from build123d import *

# Parameters (mm, degrees)
BOSS_EXTRUDE1_DEPTH      = 5
BOSS_EXTRUDE1_DEPTH_BACK = 10
SKETCH1_R                = 12.5


with BuildPart() as part:
    # Sketch1 → Boss-Extrude1 (new, two sides: drawn at the far end of the back side and taken through both)
    with BuildSketch(Plane.XY.offset(-BOSS_EXTRUDE1_DEPTH_BACK)):
        with BuildLine():
            Line((-44.88915592, -28.254421038), (-43.965658713, -46.45807859))
            ThreePointArc((-43.965658713, -46.45807859), (-28.965658713, -61.45807859), (-13.965658713, -46.45807859))
            Line((-13.965658713, -46.45807859), (-14.042670787, -44.940043234))
            Line((-14.042670787, -44.940043234), (-14.968304337, -26.694274815))
            ThreePointArc((-14.968304337, -26.694274815), (-29.72001982, -31.477043366), (-44.88915592, -28.254421038))
        make_face()
        with Locations((-28.965658713, -46.45807859)):
            Circle(SKETCH1_R, mode=Mode.SUBTRACT)
    extrude(amount=BOSS_EXTRUDE1_DEPTH + BOSS_EXTRUDE1_DEPTH_BACK)


solid = part.part
The listing builds one solid part. Answer for the finished solid, in the listing's coordinates (mm). Give positions to 0.01 mm unless a question says otherwise; leave off trailing zeros. Write each loop counter-clockwise with the first axis right and the second up, starting at its lowest first coordinate (ties: lowest second). Pieces come first, ordered by that corner, then holes. Notation, with made-up numbers: (16.5, -38) - (73.5, -38) arc R14 cw to (73.5, -27) - close; hole circle Ø11 at (32.25, 75.5). An arc over 180 degrees is marked (long way). Use a Markdown table: item, result.
1. Section C-C on y = -46 is taken. Write down the section's boundary in (x, z), plus the area to 3 significant figures.
Values follow:
| item | result |
|---|---|
| outline | (-43.99, -10) - (-41.46, -10) - (-41.46, 5) - (-43.99, 5) - close; (-16.47, -10) - (-13.99, -10) - (-13.99, 5) - (-16.47, 5) - close |
| area | 75.3 mm² |
2. For a pull along X with two mould halves and no side action, classify faces 1 (the cylindrical face through (-29.501, -31.465, -2.605)), 2 (the cylindrical face through (-22.246, -35.918, -2.605)), 3 (the flat face through (-37, -36, -10)), 4 (the cylindrical face through (-29.295, -61.454, -2.605)) as released by +X, released by -X, zero draft, split by the parting line, or undercut.
Values follow:
| item | result |
|---|---|
| face 1 | undercut |
| face 2 | undercut |
| face 3 | zero draft |
| face 4 | split by the parting line |
3. Section A-A on x = -37 is taken. Write down the section's boundary in (y, z), plus the area to 3 significant figures.
Values follow:
| item | result |
|---|---|
| outline | (-59.12, -10) - (-56.03, -10) - (-56.03, 5) - (-59.12, 5) - close; (-36.88, -10) - (-30.97, -10) - (-30.97, 5) - (-36.88, 5) - close |
| area | 135 mm² |
4. Section D-D on y = -32.5 is taken. Write down the section's boundary in (x, z), plus the area to 3 significant figures.
Values follow:
| item | result |
|---|---|
| outline | (-44.67, -10) - (-14.67, -10) - (-14.67, 5) - (-44.67, 5) - close |
| area | 450 mm² |
5. Find the intervals of material crossed by probe 1 along Y at (x, z) = (-36, 3.5); probe 2 along Y at (x, z) = (-28.5, -3.5); probe 3 along X at (y, z) = (-56.5, -7.5), in increasing order. Write a range as from..to.
Values follow:
| item | result |
|---|---|
| probe 1 | y = -59.71..-56.79, -36.13..-31.14 |
| probe 2 | y = -61.45..-58.95, -33.97..-31.39 |
| probe 3 | x = -40.11..-36.41, -21.52..-17.82 |
6. Section B-B on z = -2.5 is taken. Write down the section's boundary in (x, y), plus the area to 3 significant figures.
Values follow:
| item | result |
|---|---|
| outline | (-44.89, -28.25) - (-43.97, -46.46) arc R15 ccw to (-13.97, -46.46) - (-14.97, -26.69) arc R30 cw to start; hole circle Ø25 at (-28.97, -46.46) |
| area | 351 mm² |
7. Each of these flat-tipped pins is pushed along its axis until it touches: P1, Ø8, axis at x = -25, z = -0.5, coming from the +Y side; P2, Ø3, axis at x = -37.5, y = -43.5, coming from the +Z side; P3, Ø2, axis at x = -24.5, z = 3, coming from the +Y side; P4, Ø6, axis at y = -47, z = 1.5, coming from the -X side. Where does it stop, or does it pass through?
Values follow:
| item | result |
|---|---|
| P1 | stops at y = -29.7 |
| P2 | passes through |
| P3 | stops at y = -30.49 |
| P4 | stops at x = -44.09 |
